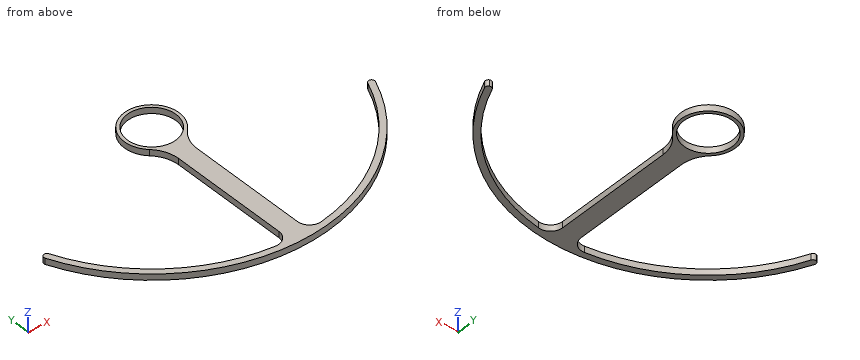
from build123d import *

# Parameters (mm, degrees)
F0_R     = 3.92
F2_DEPTH = 0.9906
F3_R     = 5.08
F4_DEPTH = 0.9906
F5_R     = 1.9460346085


with BuildPart() as f2:
    # F0 (on Top) → F2 (new body)
    with BuildSketch(Plane.XY):
        with BuildLine():
            Line((1.4986, -28.459371031), (1.4986, -4.157771302))
            ThreePointArc((1.4986, -4.157771302), (0, 4.4196), (-1.4986, -4.157771302))
            Line((-1.4986, -4.157771302), (-1.4986, -28.459371031))
            Line((-1.4986, -28.459371031), (1.4986, -28.459371031))
        make_face()
        Circle(F0_R, mode=Mode.SUBTRACT)
    extrude(amount=F2_DEPTH)

    # F3
    f3_edges = [f2.edges().sort_by_distance(p)[0] for p in [
        (1.4986, -4.157771, 0.4953),
        (-1.4986, -4.157771, 0.4953),
    ]]
    fillet(f3_edges, radius=F3_R)

    # F1 (on Top) → F4 (join)
    with BuildSketch(Plane.XY):
        with BuildLine():
            ThreePointArc((26.7401224733, -11.076121388), (26.7392931104, -10.6950451816), (26.4680773128, -10.4273480505))
            ThreePointArc((26.4680773128, -10.4273480505), (26.0909918386, -10.4298101144), (25.8249274084, -10.6970351799))
            ThreePointArc((25.8249274084, -10.6970351799), (0, -27.9527), (-25.8249274084, -10.6970351799))
            ThreePointArc((-25.8249274084, -10.6970351799), (-26.0909918386, -10.4298101144), (-26.4680773128, -10.4273480505))
            ThreePointArc((-26.4680773128, -10.4273480505), (-26.7392931104, -10.6950451816), (-26.7401224733, -11.076121388))
            ThreePointArc((-26.7401224733, -11.076121388), (0, -28.9433), (26.7401224733, -11.076121388))
        make_face()
    extrude(amount=F4_DEPTH)

    # F5
    f5_edges = [f2.edges().sort_by_distance(p)[0] for p in [
        (1.4986, -27.9125, 0.4953),
        (-1.4986, -27.9125, 0.4953),
    ]]
    fillet(f5_edges, radius=F5_R)


solid = f2.part
The model under review builds one solid part; all positions refer to its coordinate system, in mm. Round coordinates to 2 decimals unless told otherwise and drop trailing zeros. Loops run counter-clockwise (first coordinate to the right, second up) from the corner with the lowest first, then second, coordinate; pieces in that order, holes last. Notation, with made-up numbers: M 33,55.5 L 49,55.5 A34 cw 49,90.5 Z; hole C 22.25,47 d7. An arc over 180 degrees is marked long. Answer as CSV lines item,"result". Start each with the question number.
Item 1: Insertion check: P1, Ø0.5, axis at y = -20.5, z = 0.5, coming from the -X side; P2, Ø12.5, axis at x = 0, y = 0, coming from the +Z side. Each pin has a flat end and moves straight along its axis. Give the tip position at first contact, or say it passes through.
Item 2: Consider section B-B (y = 0). Write out the cut boundary in (x, z).
Item 3: Consider section C-C (z = 0.7). Write out the cut boundary in (x, y).
Item 4: Consider section D-D (y = -14.5). Write out the cut boundary in (x, z), then the cut area to 3 significant figures.
Item 5: Wall thickness on line 1 (X direction, y = -25, z = 0.1); line 2 (Y direction, x = 0, z = 0.35); line 3 (X direction, y = -14, z = 0.7): over which ranges is each line inside the solid? List them lowest first. Write a range as [from, to].
Item 6: Consider section A-A (x = 0). Write out the cut boundary in (y, z).
Answer:
1,P1,"stops at x = -20.68"
1,P2,"stops at z = 0.99"
2,outline,"M -4.42,0 L -3.92,0 L -3.92,0.99 L -4.42,0.99 Z; M 3.92,0 L 4.42,0 L 4.42,0.99 L 3.92,0.99 Z"
3,outline,"M -26.74,-11.08 A28.94 ccw 26.74,-11.08 A0.5 ccw 25.82,-10.7 A27.95 cw 3.7,-27.71 A1.95 cw 1.5,-25.78 L 1.5,-6.85 A5.08 cw 3.06,-3.19 A4.42 ccw long -3.06,-3.19 A5.08 cw -1.5,-6.85 L -1.5,-25.78 A1.95 cw -3.7,-27.71 A27.95 cw -25.82,-10.7 A0.5 ccw Z; hole C 0,0 d7.84"
4,outline,"M -25.05,0 L -23.9,0 L -23.9,0.99 L -25.05,0.99 Z; M -1.5,0 L 1.5,0 L 1.5,0.99 L -1.5,0.99 Z; M 23.9,0 L 25.05,0 L 25.05,0.99 L 23.9,0.99 Z"
4,area,"5.25 mm^2"
5,line 1,"x = [-14.58, -12.5], [-1.5, 1.5], [12.5, 14.58]"
5,line 2,"y = [-28.94, -3.92], [3.92, 4.42]"
5,line 3,"x = [-25.33, -24.19], [-1.5, 1.5], [24.19, 25.33]"
6,outline,"M -28.94,0 L -3.92,0 L -3.92,0.99 L -28.94,0.99 Z; M 3.92,0 L 4.42,0 L 4.42,0.99 L 3.92,0.99 Z"
